from build123d import *

# Parameters (mm, degrees)
SKETCH1_R           = 18
BOSS_EXTRUDE1_DEPTH = 1
SKETCH2_R           = 2
BOSS_EXTRUDE2_DEPTH = 2
SKETCH3_R           = 1
CUT_EXTRUDE1_DEPTH  = 26.632011236
CUT_EXTRUDE2_REACH  = 27.632


with BuildPart() as part:
    # Sketch1 → Boss-Extrude1 (new body)
    with BuildSketch(Plane(origin=(0, 0, 0), x_dir=(1, 0, 0), z_dir=(0, 1, 0))):
        with Locations(Location((0, 0, 0), (0, 0, 270))):
            Circle(SKETCH1_R)
    extrude(amount=BOSS_EXTRUDE1_DEPTH)

    # Sketch2 → Boss-Extrude2 (add)
    with BuildSketch(Plane.XZ):
        with Locations(Location((0, 0, 0), (0, 0, 90))):
            Circle(SKETCH2_R)
    extrude(amount=BOSS_EXTRUDE2_DEPTH)

    # Sketch3 → Cut-Extrude1 (cut, through all)
    with BuildSketch(Plane.XZ.offset(2)):
        with Locations(Location((0, 0, 0), (0, 0, 270))):
            Circle(SKETCH3_R)
    extrude(amount=-CUT_EXTRUDE1_DEPTH, mode=Mode.SUBTRACT)

    # Sketch4 → Cut-Extrude2 (cut, up to next)
    with BuildSketch(Plane(origin=(0, 1, 0), x_dir=(1, 0, 0), z_dir=(0, 1, 0)), mode=Mode.PRIVATE) as cut_extrude2_sk1:
        with BuildLine():
            Line((-3.5, 6.062177826), (-8.25, 14.289419162))
            ThreePointArc((-8.25, 14.289419162), (0, 16.5), (8.25, 14.289419162))
            Line((8.25, 14.289419162), (3.5, 6.062177826))
            ThreePointArc((3.5, 6.062177826), (0, 7), (-3.5, 6.062177826))
        make_face()
    cut_extrude2_tool1 = extrude(cut_extrude2_sk1.sketch, amount=-CUT_EXTRUDE2_REACH, mode=Mode.PRIVATE) & part.part
    # Sketch4 → Cut-Extrude2 (cut, up to next)
    with BuildSketch(Plane(origin=(0, 1, 0), x_dir=(1, 0, 0), z_dir=(0, 1, 0)), mode=Mode.PRIVATE) as cut_extrude2_sk2:
        with BuildLine():
            Line((7, 0), (16.5, 0))
            ThreePointArc((16.5, 0), (14.289419162, -8.25), (8.25, -14.289419162))
            Line((8.25, -14.289419162), (3.5, -6.062177826))
            ThreePointArc((3.5, -6.062177826), (6.062177826, -3.5), (7, 0))
        make_face()
    cut_extrude2_tool2 = extrude(cut_extrude2_sk2.sketch, amount=-CUT_EXTRUDE2_REACH, mode=Mode.PRIVATE) & part.part
    # Sketch4 → Cut-Extrude2 (cut, up to next)
    with BuildSketch(Plane(origin=(0, 1, 0), x_dir=(1, 0, 0), z_dir=(0, 1, 0)), mode=Mode.PRIVATE) as cut_extrude2_sk3:
        with BuildLine():
            Line((-3.5, -6.062177826), (-8.25, -14.289419162))
            ThreePointArc((-8.25, -14.289419162), (-14.289419162, -8.25), (-16.5, 0))
            Line((-16.5, 0), (-7, 0))
            ThreePointArc((-7, 0), (-6.062177826, -3.5), (-3.5, -6.062177826))
        make_face()
    cut_extrude2_tool3 = extrude(cut_extrude2_sk3.sketch, amount=-CUT_EXTRUDE2_REACH, mode=Mode.PRIVATE) & part.part
    add(cut_extrude2_tool1.solids().sort_by_distance((0, 1, -11.831646))[0], mode=Mode.SUBTRACT)
    add(cut_extrude2_tool2.solids().sort_by_distance((10.246506, 1, 5.915823))[0], mode=Mode.SUBTRACT)
    add(cut_extrude2_tool3.solids().sort_by_distance((-10.246506, 1, 5.915823))[0], mode=Mode.SUBTRACT)


solid = part.part
The listing builds one solid part. Answer for the finished solid, in the listing's coordinates (mm). A direction names the side the tool comes from. Coordinates: 2 decimals unless noted, no trailing zeros. Write each loop counter-clockwise with the first axis right and the second up, starting at its lowest first coordinate (ties: lowest second). Pieces come first, ordered by that corner, then holes. Notation, with made-up numbers: (-7.5, 52.5) - (7.5, 52.5) arc R22 cw to (7.5, 81.5) - close; hole circle Ø2 at (28, 61). An arc over 180 degrees is marked (long way). Return JSON: item names as keys, results as strings.
1. The part is cut by section D-D on x = 0. Determine the outline of the cut face in (y, z).
Final values:
{"outline": "(-2, -2) - (0, -2) - (0, -7) - (1, -7) - (1, -1) - (-2, -1) - close; (-2, 1) - (1, 1) - (1, 18) - (0, 18) - (0, 2) - (-2, 2) - close; (0, -18) - (1, -18) - (1, -16.5) - (0, -16.5) - close"}
2. Each of these flat-tipped pins is pushed along its axis until it touches: pin 1 Ø1.8 at (x, z) = (0, 0) entering from -Y; pin 2 Ø12 at (x, z) = (-14, 2.5) entering from -Y; pin 3 Ø11 at (x, z) = (-4.5, 0) entering from -Y. Where does it stop, or does it pass through?
Final values:
{"pin 1": "through", "pin 2": "y = 0", "pin 3": "y = -2"}
3. For a pull along Z with two mould halves and no side action, classify faces 3 (the face through (1, -2, 1)), 4 (the face through (-5.842, 0.507, 10.118)), 5 (the face through (2, -1, 0)), 6 (the face through (-1, -1, 0)) as +Z half, -Z half, draft (parallel to the pull), parting line (faces both ways), or undercut.
Final values:
{"face 3": "draft", "face 4": "undercut", "face 5": "parting line", "face 6": "undercut"}
4. The part is cut by section C-C on y = 0.55. Determine the outline of the cut face in (x, z), then the cut area to 3 significant figures.
Final values:
{"outline": "circle Ø36 at (0, 0); hole (-16.5, 0) - (-7, 0) arc R7 cw to (-3.5, 6.06) - (-8.25, 14.29) arc R16.5 ccw to start; hole (-8.25, -14.29) arc R16.5 ccw to (8.25, -14.29) - (3.5, -6.06) arc R7 cw to (-3.5, -6.06) - close; hole circle Ø2 at (0, 0); hole (3.5, 6.06) arc R7 cw to (7, 0) - (16.5, 0) arc R16.5 ccw to (8.25, 14.29) - close", "area": "664 mm^2"}
5. The part is cut by section B-B on z = -15. Determine the outline of the cut face in (x, y), then the cut area to 3 significant figures.
Final values:
{"outline": "(-9.95, 0) - (-6.87, 0) - (-6.87, 1) - (-9.95, 1) - close; (6.87, 0) - (9.95, 0) - (9.95, 1) - (6.87, 1) - close", "area": "6.15 mm^2"}
6. Which of the six approach directions +Z, -Z, +X, -X, +Y, -Y give full straight-line access (tool end or side, diameter ignored) to faces 1 (the face through (0, 1, 4)), 2 (the face through (5.908, 0.507, -10.233))?
Final values:
{"face 1": "+Z, -Z, +X, -X, +Y", "face 2": "+Y, -Y"}
7. Consider line 1 along X through (y, z) = (0.85, 7.5); line 2 along X through (y, z) = (-0.1, 0); line 3 along Z through (x, y) = (4, 0.95). Determine where each line is inside the solid, lowest interval first.
Final values:
{"line 1": "-16.36 to -14.7, -4.33 to 4.33, 14.7 to 16.36", "line 2": "-2 to -1, 1 to 2", "line 3": "-17.55 to -16.01, -6.93 to 5.74, 6.93 to 17.55"}
8. The part is cut by section A-A on x = -10. Determine the outline of the cut face in (y, z).
Final values:
{"outline": "(0, -14.97) - (1, -14.97) - (1, 0) - (0, 0) - close; (0, 13.12) - (1, 13.12) - (1, 14.97) - (0, 14.97) - close"}
